The model under review builds one solid part; all positions refer to its coordinate system, in mm. Face numbers are marked on the shaded views. A direction names the side the tool comes from. Coordinates: 2 decimals unless noted, no trailing zeros. Order: outer loops, then holes, each group sorted by start corner. A loop starts at its lowest first (then second) coordinate and runs counter-clockwise, first axis right, second up. Notation, with made-up numbers: M -31,45 L 8,45 A30 cw 8,83 Z; hole C -3,11 d4. An arc over 180 degrees is marked long. Answer in a Markdown table with one row per item.
from build123d import *

# Parameters (mm, degrees)
SKETCH1_W                = 15
SKETCH1_H                = 13
SKETCH1_W_2              = 12.1
SKETCH1_H_2              = 10.1
BOSS_EXTRUDE1_DEPTH      = 7
BOSS_EXTRUDE2_DEPTH      = 17
BOSS_EXTRUDE2_DEPTH_BACK = 7
SKETCH2_W                = 5.674885541
SKETCH2_H                = 3
BOSS_EXTRUDE3_DEPTH      = 2
FILLET1_START            = -4.744281145
FILLET1_DEPTH            = 3.685449278
FILLET1_START_2          = 7.64136832
FILLET1_2_DEPTH          = 2.564121617
FILLET1_START_3          = 5.430604396
FILLET1_3_DEPTH          = 2.210763824
FILLET1_START_4          = -1.058831867
FILLET1_4_DEPTH          = 1.089436263
FILLET1_START_5          = -8
FILLET1_5_DEPTH          = 6


with BuildPart() as part:
    # Sketch1 → Boss-Extrude1 (new body)
    with BuildSketch(Plane.XY):
        with Locations((2.705489937, 9.533064254)):
            Rectangle(SKETCH1_W, SKETCH1_H)
        with Locations((2.705489937, 9.533064254)):
            Rectangle(SKETCH1_W_2, SKETCH1_H_2, mode=Mode.SUBTRACT)
    extrude(amount=BOSS_EXTRUDE1_DEPTH)

    # Sketch2 → Boss-Extrude2 (add, two sides: drawn at the far end of the back side and taken through both)
    with BuildSketch(Plane(origin=(0, 0, 0), x_dir=(-1, 0, 0), z_dir=(0, 0, -1)).offset(-BOSS_EXTRUDE2_DEPTH_BACK)):
        with Locations((-7.368047167, 17.22155756)):
            Rectangle(SKETCH2_W, SKETCH2_H)
        with Locations((1.906838375, 17.22155756)):
            Rectangle(SKETCH2_W, SKETCH2_H)
    extrude(amount=BOSS_EXTRUDE2_DEPTH + BOSS_EXTRUDE2_DEPTH_BACK)

    # Sketch3 → Boss-Extrude3 (add)
    with BuildSketch(Plane(origin=(0, 0, 0), x_dir=(-1, 0, 0), z_dir=(0, 0, -1))):
        with BuildLine():
            Line((-10.205489937, 15.72155756), (-5.430604396, 15.72155756))
            Line((-5.430604396, 15.72155756), (-5.430604396, 13.72345972))
            ThreePointArc((-5.430604396, 13.72345972), (-7.053489061, 11.951422257), (-7.64136822, 9.62155756))
            Line((-7.64136822, 9.62155756), (-7.64136822, 3.033064254))
            Line((-7.64136822, 3.033064254), (-10.205489937, 3.033064254))
            Line((-10.205489937, 3.033064254), (-10.205489937, 9.62155756))
            Line((-10.205489937, 9.62155756), (-10.205489937, 13.72345972))
            Line((-10.205489937, 13.72345972), (-10.205489937, 15.72155756))
        make_face()
        with BuildLine():
            Line((4.744281145, 15.72155756), (4.744281145, 13.72345972))
            Line((4.744281145, 13.72345972), (4.744281145, 9.62155756))
            Line((4.744281145, 9.62155756), (4.744281145, 3.033064254))
            Line((4.744281145, 3.033064254), (2.180159427, 3.033064254))
            Line((2.180159427, 3.033064254), (2.180159427, 9.62155756))
            ThreePointArc((2.180159427, 9.62155756), (1.592280269, 11.951422257), (-0.030604396, 13.72345972))
            Line((-0.030604396, 13.72345972), (-0.030604396, 15.72155756))
            Line((-0.030604396, 15.72155756), (4.744281145, 15.72155756))
        make_face()
    extrude(amount=BOSS_EXTRUDE3_DEPTH)

    # Fillet1: read off the stored shape, not the designer's step
    # Fillet1 outline → Fillet1 (add)
    with BuildSketch(Plane.YZ.offset(FILLET1_START)):
        with BuildLine():
            ThreePointArc((9.72155756, -2), (13.964198247, -3.757359313), (15.72155756, -8))
            Line((15.72155756, -8), (15.72155756, -2))
            Line((15.72155756, -2), (9.72155756, -2))
        make_face()
    extrude(amount=FILLET1_DEPTH)

    # Fillet1 2 outline → Fillet1 2 (add)
    with BuildSketch(Plane.YZ.offset(FILLET1_START_2)):
        with BuildLine():
            ThreePointArc((9.72155756, -2), (13.964198247, -3.757359313), (15.72155756, -8))
            Line((15.72155756, -8), (15.72155756, -2))
            Line((15.72155756, -2), (9.72155756, -2))
        make_face()
    extrude(amount=FILLET1_2_DEPTH)

    # Fillet1 3 outline → Fillet1 3 (add)
    with BuildSketch(Plane.YZ.offset(FILLET1_START_3)):
        with BuildLine():
            ThreePointArc((9.72155756, -2), (13.964198247, -3.757359313), (15.72155756, -8))
            Line((15.72155756, -8), (15.72155756, -2))
            Line((15.72155756, -2), (9.72155756, -2))
        make_face()
    extrude(amount=FILLET1_3_DEPTH)

    # Fillet1 4 outline → Fillet1 4 (add)
    with BuildSketch(Plane.YZ.offset(FILLET1_START_4)):
        with BuildLine():
            ThreePointArc((9.72155756, -2), (13.964198247, -3.757359313), (15.72155756, -8))
            Line((15.72155756, -8), (15.72155756, -2))
            Line((15.72155756, -2), (9.72155756, -2))
        make_face()
    extrude(amount=FILLET1_4_DEPTH)

    # Fillet1 5 outline → Fillet1 5 (cut)
    with BuildSketch(Plane.XY.offset(FILLET1_START_5)):
        with BuildLine():
            Line((7.64136822, 8), (7.64136822, 9.62155756))
            ThreePointArc((7.64136822, 9.62155756), (7.053489061, 11.951422256), (5.430604396, 13.72345972))
            Line((5.430604396, 13.72345972), (5.430604396, 8))
            Line((5.430604396, 8), (7.64136822, 8))
        make_face()
        with BuildLine():
            Line((-2.180159426, 8), (0.030604396, 8))
            Line((0.030604396, 8), (0.030604396, 13.72345972))
            ThreePointArc((0.030604396, 13.72345972), (-1.592280269, 11.951422257), (-2.180159427, 9.62155756))
            Line((-2.180159427, 9.62155756), (-2.180159426, 8))
        make_face()
    extrude(amount=FILLET1_5_DEPTH, mode=Mode.SUBTRACT)


solid = part.part
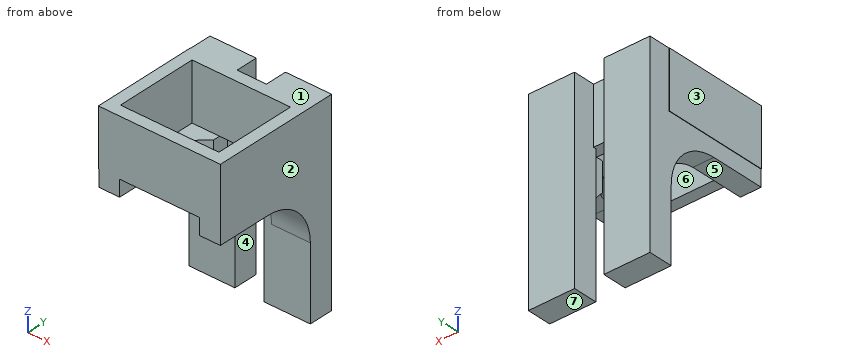
(1) Take a section at D-D (y = 12). Write out the cut boundary in (x, z), then the cut area to 3 significant figures.
Report:
| item | result |
|---|---|
| outline | M -4.79,0 L -4.74,0 L -4.74,-2.45 L -1.57,-2.45 L -1.57,0 L -3.34,0 L -3.34,7 L -4.79,7 Z; M 7.03,-2.45 L 10.21,-2.45 L 10.21,7 L 8.76,7 L 8.76,0 L 7.03,0 Z |
| area | 35.9 mm^2 |
(2) Take a section at A-A (z = -8.75). Write out the cut boundary in (x, y).
Report:
| item | result |
|---|---|
| outline | M -4.74,15.72 L 0.93,15.72 L 0.93,18.72 L -4.74,18.72 Z; M 4.53,15.72 L 10.21,15.72 L 10.21,18.72 L 4.53,18.72 Z |
(3) To check wall thickness, follow line 1 (Y direction, x = 1, z = 4); line 2 (Y direction, x = 5, z = 6.25); line 3 (X direction, y = 13.5, z = 3). State the ranges of each line that lie inside material, in increasing order. Write a range as [from, to].
Report:
| item | result |
|---|---|
| line 1 | [3.03, 4.48], [14.58, 16.03] |
| line 2 | [3.03, 4.48], [14.58, 18.72] |
| line 3 | [-4.79, -3.34], [8.76, 10.21] |
(4) Take a section at C-C (z = 4.5). Write out the cut boundary in (x, y), then the cut area to 3 significant figures.
Report:
| item | result |
|---|---|
| outline | M -4.79,3.03 L 10.21,3.03 L 10.21,18.72 L 4.53,18.72 L 4.53,16.03 L 0.93,16.03 L 0.93,18.72 L -4.74,18.72 L -4.74,16.03 L -4.79,16.03 Z; hole M -3.34,4.48 L 8.76,4.48 L 8.76,14.58 L -3.34,14.58 Z |
| area | 103 mm^2 |
(5) The part is to be moulded in two halves that separate along X. For the marked faces 1, 2, 3 and 4, say which applies: +X half, -X half, draft (parallel to the pull), parting line (faces both ways), or undercut.
Report:
| item | result |
|---|---|
| face 1 | draft |
| face 2 | +X half |
| face 3 | -X half |
| face 4 | undercut |
(6) Take a section at B-B (x = 1.5). Write out the cut boundary in (y, z), then the cut area to 3 significant figures.
Report:
| item | result |
|---|---|
| outline | M 3.03,0 L 4.48,0 L 4.48,7 L 3.03,7 Z; M 14.58,0 L 16.03,0 L 16.03,7 L 14.58,7 Z |
| area | 20.3 mm^2 |
(7) Machinability: for the marked faces 5, 6 and 7, which of the approach directions +Z, -Z, +X, -X, +Y, -Y give a long, thin tool a straight path to every point of the face, cutting with its end or side? Answer none if there is none.
Report:
| item | result |
|---|---|
| face 5 | -Z, +X, -X, -Y |
| face 6 | +Z |
| face 7 | -Z, +X, -X, +Y, -Y |
(8) Insertion check: P1, Ø8, axis at x = -3, y = 8.5, coming from the -Z side; P2, Ø0.9, axis at y = 17, z = -8.5, coming from the -X side; P3, Ø1.3, axis at x = 9, y = 7.5, coming from the -Z side. Each pin has a flat end and moves straight along its axis. Give the tip position at first contact, or say it passes through.
Report:
| item | result |
|---|---|
| P1 | z = -2.68 |
| P2 | x = -4.74 |
| P3 | z = -2 |
